Geometry check sheet. Reference: drawing and pictorial views, mm from the part's lowest x, y, z. Give positions to 0.01 mm unless a question says otherwise; leave off trailing zeros. Order: outer loops, then holes, each group sorted by start corner. A loop starts at its lowest first (then second) coordinate and runs counter-clockwise, first axis right, second up.
Item 1: Material ranges on line 1 along Z through (x, y) = (4.5, 76) (1 decimal); line 2 along Y through (x, z) = (3, 114.5) (1 decimal); line 3 along Z through (x, y) = (4, 95) (1 decimal), recorded low to high.
Item 2: Sectioned sample at B-B on z = 17. Record the boundary of the cut face in (x, y).
Item 3: Gauge pin test, flat ends, axial feed: P1, Ø1.5, axis at x = 3.5, z = 55, coming from the +Y side; P2, Ø1, axis at x = 1, z = 52, coming from the +Y side. Record the tip position at first contact, or that the pin passes through.
Item 4: Sectioned sample at A-A on z = 114. Record the boundary of the cut face in (x, y) (1 decimal).
Item 5: Sectioned sample at C-C on x = 2.5. Count the separate pieces of the cut face and the enclosed holes in it, and give its area (3 significant figures).
Item 6: Sectioned sample at D-D on z = 42.5. Record the boundary of the cut face in (x, y).
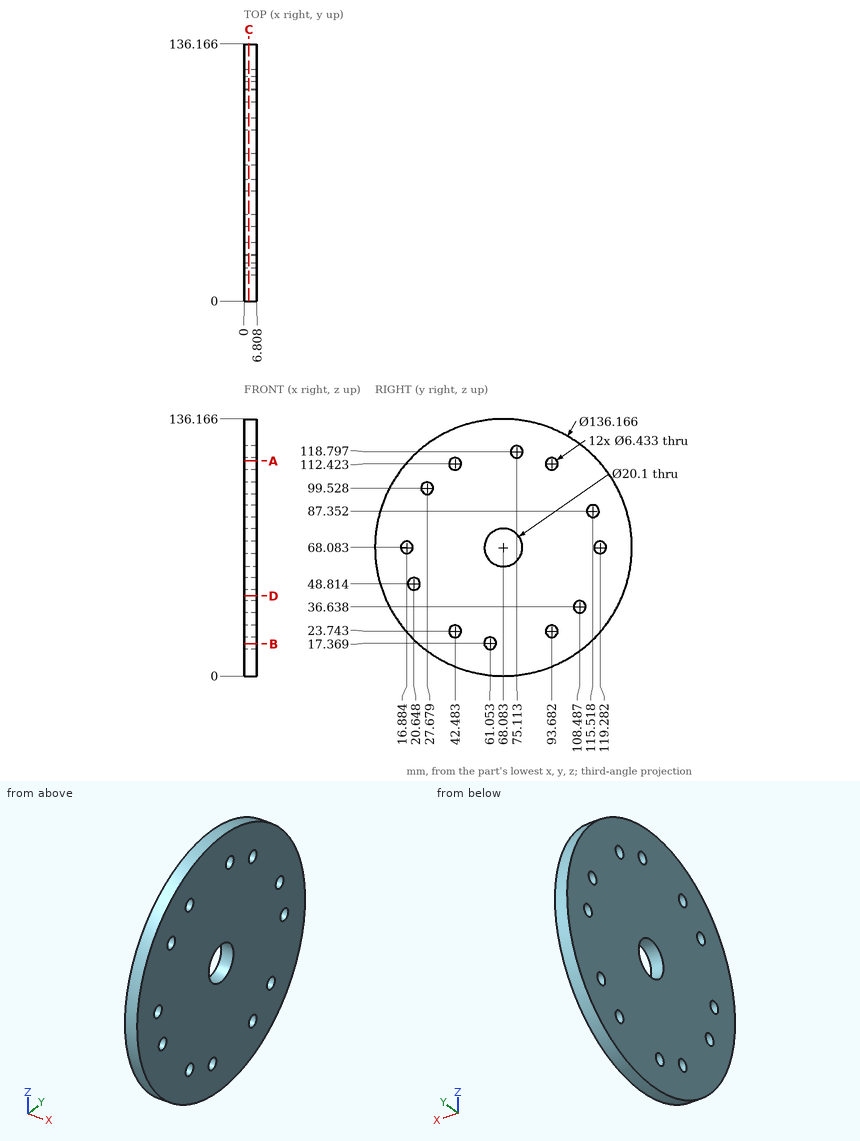
Report:
1. line 1: z = 0.5 to 61.9, 74.3 to 115.7, 121.9 to 135.7
1. line 2: y = 18.3 to 40, 44.9 to 91.2, 96.1 to 117.9
1. line 3: z = 5.5 to 20.8, 26.7 to 109.5, 115.4 to 130.6
2. outline: (0, 23.07) - (6.81, 23.07) - (6.81, 57.86) - (0, 57.86) - close; (0, 64.25) - (6.81, 64.25) - (6.81, 113.09) - (0, 113.09) - close
3. P1: stops at y = 135.04
3. P2: stops at y = 134.36
4. outline: (0, 17.8) - (6.8, 17.8) - (6.8, 39.7) - (0, 39.7) - close; (0, 45.3) - (6.8, 45.3) - (6.8, 90.9) - (0, 90.9) - close; (0, 96.5) - (6.8, 96.5) - (6.8, 118.4) - (0, 118.4) - close
5. separate pieces: 1
5. enclosed holes: 13
5. area: 13,900 mm2
6. outline: (0, 4.99) - (6.81, 4.99) - (6.81, 131.18) - (0, 131.18) - close
